```python
from build123d import *

# Parameters (mm, degrees)
SKETCH_1_R      = 2
SKETCH_1_R_2    = 1.5
SKETCH_1_W      = 5.05
SKETCH_1_H      = 2.05
EXTRUDE_1_DEPTH = 2


with BuildPart() as part:
    # 草图1 → 凸台-拉伸1 (new body)
    with BuildSketch(Plane.XY):
        with BuildLine():
            Line((317.453360513, 294.462931603), (319.953360513, 294.462931603))
            Line((319.953360513, 294.462931603), (319.953360513, 275.962931603))
            Line((319.953360513, 275.962931603), (279.953360513, 255.962931603))
            ThreePointArc((279.953360513, 255.962931603), (251.095061372, 225.984664155), (220.040259237, 253.681184024))
            ThreePointArc((220.040259237, 253.681184024), (219.19036683, 255.554039999), (217.334030317, 256.439433332))
            add(Edge.make_bspline(
                [(217.334030317, 256.439433332), (215.548727104, 256.609856683), (206.547632182, 255.661407624), (194.456958912, 237.242452466), (194.688078584, 213.970775709), (179.953360513, 219.413055772)],
                knots=[0.04025352, 0.04025352, 0.04025352, 0.04025352, 0.124939279, 0.47725999, 1, 1, 1, 1], degree=3))
            Line((179.953360513, 219.413055772), (179.953360513, 224.462931603))
            Line((179.953360513, 224.462931603), (177.953360513, 224.462931603))
            Line((177.953360513, 224.462931603), (177.953360513, 229.462931603))
            Line((177.953360513, 229.462931603), (179.953360513, 229.462931603))
            Line((179.953360513, 229.462931603), (179.953360513, 234.462931603))
            Line((179.953360513, 234.462931603), (177.953360513, 234.462931603))
            Line((177.953360513, 234.462931603), (177.953360513, 239.462931603))
            Line((177.953360513, 239.462931603), (179.953360513, 239.462931603))
            Line((179.953360513, 239.462931603), (179.953360513, 254.462931603))
            Line((179.953360513, 254.462931603), (182.453360513, 254.462931603))
            Line((182.453360513, 254.462931603), (182.453360513, 252.962931602))
            Line((182.453360513, 252.962931602), (185.053360513, 252.962931602))
            Line((185.053360513, 252.962931602), (185.053360513, 254.462931603))
            Line((185.053360513, 254.462931603), (188.053360513, 254.462931603))
            Line((188.053360513, 254.462931603), (188.053360513, 257.462931602))
            Line((188.053360513, 257.462931602), (185.053360513, 257.462931602))
            Line((185.053360513, 257.462931602), (185.053360513, 258.962931602))
            Line((185.053360513, 258.962931602), (182.453360513, 258.962931602))
            Line((182.453360513, 258.962931602), (182.453360513, 257.462931603))
            Line((182.453360513, 257.462931603), (179.953360513, 257.462931603))
            Line((179.953360513, 257.462931603), (179.953360513, 294.462931603))
            Line((179.953360513, 294.462931603), (182.453360513, 294.462931603))
            Line((182.453360513, 294.462931603), (182.453360513, 292.962931603))
            Line((182.453360513, 292.962931603), (185.053360513, 292.962931603))
            Line((185.053360513, 292.962931603), (185.053360513, 294.462931603))
            Line((185.053360513, 294.462931603), (188.053360513, 294.462931603))
            Line((188.053360513, 294.462931603), (188.053360513, 297.462931603))
            Line((188.053360513, 297.462931603), (185.053360513, 297.462931603))
            Line((185.053360513, 297.462931603), (185.053360513, 298.962931603))
            Line((185.053360513, 298.962931603), (182.453360513, 298.962931603))
            Line((182.453360513, 298.962931603), (182.453360513, 297.462931603))
            Line((182.453360513, 297.462931603), (179.953360513, 297.462931603))
            Line((179.953360513, 297.462931603), (179.953360513, 312.462931603))
            Line((179.953360513, 312.462931603), (177.953360513, 312.462931603))
            Line((177.953360513, 312.462931603), (177.953360513, 317.462931603))
            Line((177.953360513, 317.462931603), (179.953360513, 317.462931603))
            Line((179.953360513, 317.462931603), (179.953360513, 322.462931603))
            Line((179.953360513, 322.462931603), (177.953360513, 322.462931603))
            Line((177.953360513, 322.462931603), (177.953360513, 327.462931603))
            Line((177.953360513, 327.462931603), (179.953360513, 327.462931603))
            Line((179.953360513, 327.462931603), (179.953360513, 338.462931603))
            Line((179.953360513, 338.462931603), (319.953360513, 338.462931603))
            Line((319.953360513, 338.462931603), (319.953360513, 327.462931603))
            Line((319.953360513, 327.462931603), (321.953360513, 327.462931603))
            Line((321.953360513, 327.462931603), (321.953360513, 322.462931603))
            Line((321.953360513, 322.462931603), (319.953360513, 322.462931603))
            Line((319.953360513, 322.462931603), (319.953360513, 317.462931603))
            Line((319.953360513, 317.462931603), (321.953360513, 317.462931603))
            Line((321.953360513, 317.462931603), (321.953360513, 312.462931603))
            Line((321.953360513, 312.462931603), (319.953360513, 312.462931603))
            Line((319.953360513, 312.462931603), (319.953360513, 297.462931603))
            Line((319.953360513, 297.462931603), (317.453360513, 297.462931603))
            Line((317.453360513, 297.462931603), (317.453360513, 298.962931603))
            Line((317.453360513, 298.962931603), (314.853360513, 298.962931603))
            Line((314.853360513, 298.962931603), (314.853360513, 297.462931603))
            Line((314.853360513, 297.462931603), (311.853360513, 297.462931603))
            Line((311.853360513, 297.462931603), (311.853360513, 294.462931603))
            Line((311.853360513, 294.462931603), (314.853360513, 294.462931603))
            Line((314.853360513, 294.462931603), (314.853360513, 292.962931603))
            Line((314.853360513, 292.962931603), (317.453360513, 292.962931603))
            Line((317.453360513, 292.962931603), (317.453360513, 294.462931603))
        make_face()
        with Locations((249.953360513, 255.962931603)):
            Circle(SKETCH_1_R, mode=Mode.SUBTRACT)
        with Locations((229.953360513, 335.462931603)):
            Circle(SKETCH_1_R_2, mode=Mode.SUBTRACT)
        with Locations((269.953360513, 335.462931603)):
            Circle(SKETCH_1_R_2, mode=Mode.SUBTRACT)
        with Locations((229.953360513, 295.962931603)):
            Circle(SKETCH_1_R, mode=Mode.SUBTRACT)
        with Locations((269.953360513, 295.962931603)):
            Circle(SKETCH_1_R, mode=Mode.SUBTRACT)
        with Locations((288.953360513, 335.462931603)):
            Rectangle(SKETCH_1_W, SKETCH_1_H, mode=Mode.SUBTRACT)
        with Locations((298.953360513, 335.462931603)):
            Rectangle(SKETCH_1_W, SKETCH_1_H, mode=Mode.SUBTRACT)
        with Locations((200.953360513, 335.462931603)):
            Rectangle(SKETCH_1_W, SKETCH_1_H, mode=Mode.SUBTRACT)
        with Locations((210.953360513, 335.462931603)):
            Rectangle(SKETCH_1_W, SKETCH_1_H, mode=Mode.SUBTRACT)
    extrude(amount=EXTRUDE_1_DEPTH)


solid = part.part
```
Verification items for the finished model (mm, model axes). Round coordinates to 2 decimals unless told otherwise and drop trailing zeros. Write each loop counter-clockwise with the first axis right and the second up, starting at its lowest first coordinate (ties: lowest second). Pieces come first, ordered by that corner, then holes.
1. Section check A-A on y = 309.5. Enter the section's corners in (x, z), plus the area to 3 significant figures.
2. Section check C-C on z = 1.05. State how many separate pieces and enclosed holes the cut face has, plus the area to 3 significant figures.
3. Gauge pin test, flat ends, axial feed: P1, Ø1, axis at x = 181.5, z = 1, coming from the -Y side; P2, Ø1, axis at x = 288, z = 1.5, coming from the -Y side; P3, Ø2.5, axis at x = 269.95, y = 335.46, coming from the -Z side; P4, Ø1, axis at y = 301.5, z = 0.5, coming from the -X side. Record the tip position at first contact, or that the pin passes through.
4. Draft check along X on faces 1 (the flat face through (300.23, 266.1, 0.99)), 2 (the flat face through (251, 291, 2)), 3 (the cylindrical face through (231.03, 297.65, 0.99)). Enter one of: +X half, -X half, draft (parallel to the pull), parting line (faces both ways), or undercut.
5. Scan lines: L1, parallel to Y at x = 270, z = 1.6; L2, parallel to Y at x = 187, z = 1.4; L3, parallel to X at y = 276.5, z = 0.3. Record each from-to range of solid material in increasing order.
6. Section check B-B on x = 238.5. Enter the section's corners in (y, z), plus the area to 3 significant figures.
Answer:
1. outline: (179.95, 0) - (319.95, 0) - (319.95, 2) - (179.95, 2) - close
1. area: 280 mm2
2. separate pieces: 1
2. enclosed holes: 9
2. area: 13,100 mm2
3. P1: stops at y = 218.75
3. P2: stops at y = 259.74
3. P3: passes through
3. P4: stops at x = 179.95
4. face 1: +X half
4. face 2: draft
4. face 3: undercut
5. L1: y = 233.64 to 293.96, 297.96 to 333.96, 336.96 to 338.46
5. L2: y = 218.27 to 254.46, 257.46 to 294.46, 297.46 to 338.46
5. L3: x = 179.95 to 319.95
6. outline: (228.24, 0) - (338.46, 0) - (338.46, 2) - (228.24, 2) - close
6. area: 220 mm2
